Autodesk Inventor part; units mm, degrees
ref_plane "YZ Plane" through (0, 0, 0) normal (1, 0, 0) x (0, 1, 0)
ref_plane "XZ Plane" through (0, 0, 0) normal (0, 1, 0) x (-1, 0, 0)
ref_plane "XY Plane" through (0, 0, 0) normal (0, 0, 1) x (1, 0, 0)
sketch "Sketch1" plane through (0, 0, 0) normal (0, 0, 1) x (1, 0, 0)
  circle A0 centre (0, 0) radius 28
  line L0 (-27.5, 5.5) -> (27.5, 5.5)
  line L1 (27.5, 5.5) -> (27.5, 4)
  line L2 (27.5, 4) -> (-27.5, 4)
  line L3 (-27.5, 4) -> (-27.5, 5.5)
  line L4 (-27.7128, 4) -> (27.7128, 4)
  line L5 (-14.7128, 4) -> (-14.7128, -1)
  line L6 (-14.7128, -1) -> (-25.7488, -11)
  line L7 (-27.5, 4.75) -> (-21.5, 4.75)
  dimension "d0" = 56
  dimension "d1" = 55
  dimension "d2" = 1.5
  dimension "d3" = 27.5
  dimension "d4" = 4
  dimension "d5" = 4
  dimension "d6" = 5
  dimension "d7" = 13
  dimension "d8" = 15
  dimension "d12" = 6
  dimension "d13" = 6.2128
extrude "Extrusion1" add sketch "Sketch1" along normal mid plane 15 contours A0 L4 L2 L5 L6 picked at (-22.5928, -6.0493)
sketch "Sketch2" plane through (-27.7128, 4, 7.5) normal (0, 1, 0) x (1, 0, 0)
  line L0 (6.213, 11.8879) -> (10.013, 9.6939)
  line L1 (10.013, 9.6939) -> (10.013, 5.3061)
  line L2 (10.013, 5.3061) -> (6.213, 3.1121)
  line L3 (6.213, 3.1121) -> (2.413, 5.3061)
  line L4 (2.413, 5.3061) -> (2.413, 9.6939)
  line L5 (2.413, 9.6939) -> (6.213, 11.8879)
  line L6 (0, 15) -> (0, 0)
  line L7 (13, 15) -> (13, 0)
  line L8 (13, 7.5) -> (0, 7.5)
  point P0 (27.7128, 7.5)
  point P1 (6.213, 7.5)
  dimension "d14" = 6.213
  dimension "d15" = 0
  dimension "d16" = 7.6
extrude "Extrusion2" cut sketch "Sketch2" against normal blind 3
sketch "Sketch3" plane through (-27.7128, 1, 7.5) normal (0, 1, 0) x (1, 0, 0)
  circle A0 centre (6.213, 7.5) radius 1.75
  point P0 (27.7128, 7.5)
  dimension "d19" = 3.5
extrude "Extrusion3" cut sketch "Sketch3" against normal blind 10
properties part number "Soporte placa"
Model file for the job. Use its own axes, mm. A direction names the side the tool comes from. Round coordinates to 2 decimals unless told otherwise and drop trailing zeros. Write each loop counter-clockwise with the first axis right and the second up, starting at its lowest first coordinate (ties: lowest second). Pieces come first, ordered by that corner, then holes. Notation, with made-up numbers: (-30.5, 83.5) - (15.5, 83.5) arc R34 ccw to (15.5, 113.5) - close; hole circle Ø9 at (71.25, -22). An arc over 180 degrees is marked (long way). Use CSV: the item, a comma, the result in double quotes. Start each with the question number.
Item 1: Band-saw the part on A-A (z = 0.5). Write the cut outline in (x, y), and give its area (3 significant figures).
Item 2: Band-saw the part on D-D (x = -19). Write the cut outline in (y, z), and give its area (3 significant figures).
Item 3: Band-saw the part on B-B (y = -4.5). Write the cut outline in (x, z), and give its area (3 significant figures).
Item 4: Drill centre lines: L1, parallel to Z at x = -20.25, y = 0.25; L2, parallel to Z at x = -24.5, y = 3; L3, parallel to X at y = -3, z = 0. Where is each one in solid material? Low to high. Write a range as [from, to].
Item 5: Pin check, flat tips, straight feed: P1, Ø2, axis at x = -21.5, z = 0, coming from the +Y side; P2, Ø4, axis at x = -21, z = 5, coming from the -Y side; P3, Ø6, axis at y = -9, z = -6, coming from the +X side; P4, Ø0.9, axis at y = 3, z = 1, coming from the -X side. Stop position of each tip, or through.
Item 6: Band-saw the part on C-C (z = 2.5). Write the cut outline in (x, y), and give its area (3 significant figures).
Item 7: Tool access for faces 1 (the face through (-23.426, 2.521, -3.276)), 2 (the face through (-23, -2, -7.5)): list every direction of +Z, -Z, +X, -X, +Y, -Y with a clear straight run to the whole face (end or side of a thin tool).
Item 8: Two-plate mould, pull along X, no slides. Class faces 3 (the face through (-23.248, -2.726, -0.077)), 4 (the face through (-23, -2, 7.5)), 5 (the face through (-19.573, 2.521, 3.276)), 6 (the face through (-14.713, 2, 0)): released by +X, released by -X, zero draft, split by the parting line, or undercut.
Checked values:
1,outline,"(-27.71, 4) arc R28 ccw to (-25.75, -11) - (-23.18, -8.67) - (-23.18, 1) - (-25.3, 1) - (-25.3, 4) - close; (-19.82, -5.63) - (-14.71, -1) - (-14.71, 4) - (-17.7, 4) - (-17.7, 1) - (-19.82, 1) - close"
1,area,"85.5 mm²"
2,outline,"(-4.88, -7.5) - (4, -7.5) - (4, -2.94) - (1, -2.94) - (1, 2.94) - (4, 2.94) - (4, 7.5) - (-4.88, 7.5) - close"
2,area,"116 mm²"
3,outline,"(-27.64, -7.5) - (-18.58, -7.5) - (-18.58, 7.5) - (-27.64, 7.5) - close; hole circle Ø3.5 at (-21.5, 0)"
3,area,"126 mm²"
4,L1,"z = [-7.5, -1.22], [1.22, 7.5]"
4,L2,"z = [-7.5, -2.66], [2.66, 7.5]"
4,L3,"x = [-27.84, -23.25], [-19.75, -16.92]"
5,P1,"passes through"
5,P2,"stops at y = -8.51"
5,P3,"stops at x = -20.23"
5,P4,"stops at x = -27.88"
6,outline,"(-27.71, 4) arc R28 ccw to (-25.75, -11) - (-14.71, -1) - (-14.71, 4) - (-18.23, 4) - (-18.23, 1) - (-24.77, 1) - (-24.77, 4) - close"
6,area,"116 mm²"
7,face 1,"+Y"
7,face 2,"-Z, +X, -X, +Y, -Y"
8,face 3,"undercut"
8,face 4,"zero draft"
8,face 5,"undercut"
8,face 6,"released by +X"
